Here's the drawing with two shaded views (mm, measured from the low corner). I have some questions. Coordinates: 2 decimals unless noted, no trailing zeros. Write each loop counter-clockwise with the first axis right and the second up, starting at its lowest first coordinate (ties: lowest second). Pieces come first, ordered by that corner, then holes.
Item 1: I'm going to push flat-ended pins straight in: pin 1 Ø3 at (y, z) = (32.5, 1.5) entering from +X; pin 2 Ø1.2 at (y, z) = (40, 78.25) entering from +X; pin 3 Ø2 at (x, y) = (5.5, 28.5) entering from -Z. Where does each tip first touch, or does it pass through?
Item 2: If we section it at D-D (y = 34.5): Please give me the cut outline in (x, z).
Item 3: If I drill on line 1 (Z direction, x = 3.75, y = 40); line 2 (Y direction, x = 1.7, z = 78.25); line 3 (Z direction, x = 6.75, y = 45), over which ranges is the centre line in solid material (lowest first)?
Item 4: If we section it at C-C (z = 78.25): Please give me the cut outline in (x, y).
Item 5: If we section it at B-B (y = 40): Please give me the cut outline in (x, z), then the cut area to 3 significant figures.
Item 6: If we section it at A-A (x = 6.75): Please give me the cut outline in (y, z), then the cut area to 4 significant figures.
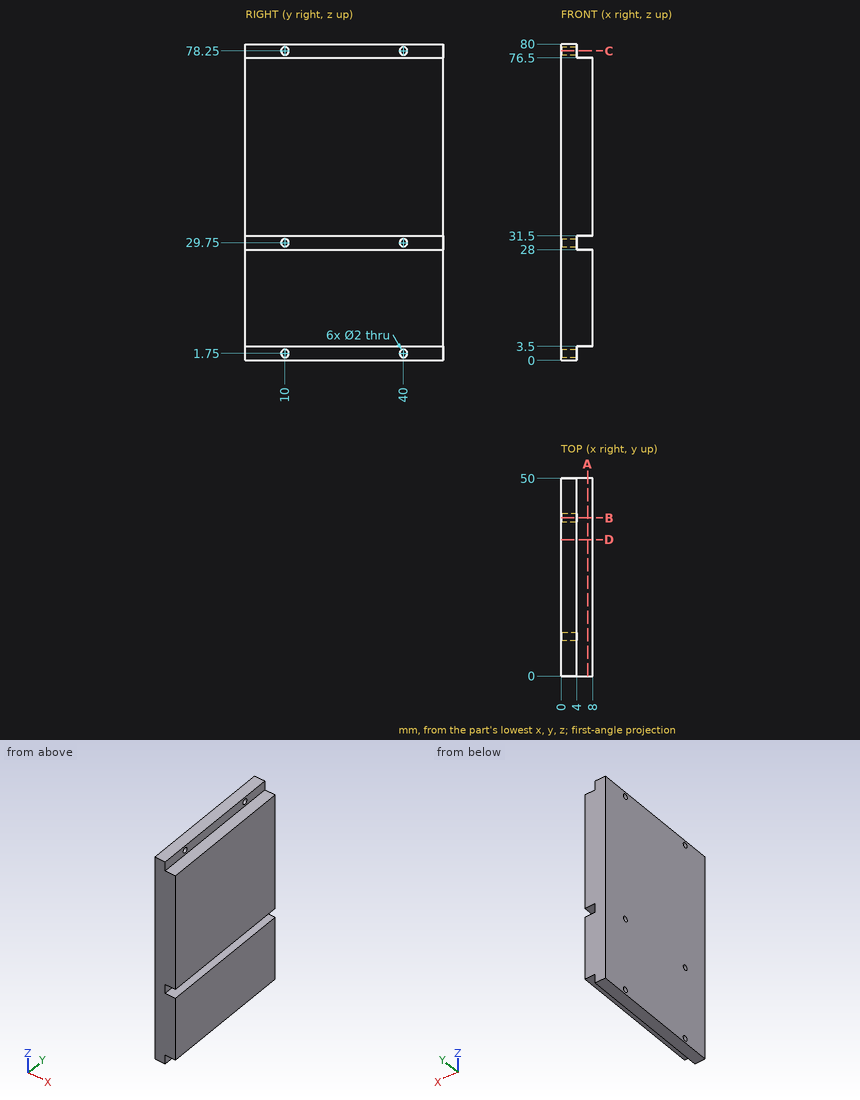
Answer list:
1. pin 1: stops at x = 4
1. pin 2: passes through
1. pin 3: stops at z = 3.5
2. outline: (0, 0) - (4, 0) - (4, 3.5) - (8, 3.5) - (8, 28) - (4, 28) - (4, 31.5) - (8, 31.5) - (8, 76.5) - (4, 76.5) - (4, 80) - (0, 80) - close
3. line 1: z = 0 to 0.75, 2.75 to 28.75, 30.75 to 77.25, 79.25 to 80
3. line 2: y = 0 to 9, 11 to 39, 41 to 50
3. line 3: z = 3.5 to 28, 31.5 to 76.5
4. outline: (0, 0) - (4, 0) - (4, 9) - (0, 9) - close; (0, 11) - (4, 11) - (4, 39) - (0, 39) - close; (0, 41) - (4, 41) - (4, 50) - (0, 50) - close
5. outline: (0, 0) - (4, 0) - (4, 0.75) - (0, 0.75) - close; (0, 2.75) - (4, 2.75) - (4, 3.5) - (8, 3.5) - (8, 28) - (4, 28) - (4, 28.75) - (0, 28.75) - close; (0, 30.75) - (4, 30.75) - (4, 31.5) - (8, 31.5) - (8, 76.5) - (4, 76.5) - (4, 77.25) - (0, 77.25) - close; (0, 79.25) - (4, 79.25) - (4, 80) - (0, 80) - close
5. area: 574 mm2
6. outline: (0, 3.5) - (50, 3.5) - (50, 28) - (0, 28) - close; (0, 31.5) - (50, 31.5) - (50, 76.5) - (0, 76.5) - close
6. area: 3,475 mm2
